CAD build for the part. Positions are in the model's coordinates, mm. A direction names the side the tool comes from. Give positions to 0.01 mm unless a question says otherwise; leave off trailing zeros. Write each loop counter-clockwise with the first axis right and the second up, starting at its lowest first coordinate (ties: lowest second). Pieces come first, ordered by that corner, then holes. Notation, with made-up numbers: (6.5, -32) - (10.5, -32) arc R13 cw to (10.5, -16) - close; hole circle Ø4 at (72.25, 53.25). An arc over 180 degrees is marked (long way). Put each result on its own line as item: value. Start each with the question number.
1. Cut at A-A on y = 28.5. List the corners of the cut face in (x, z), and give its area (3 significant figures).
2. Cut at C-C on x = -20. List the corners of the cut face in (y, z).
3. Cut at B-B on x = 28. List the corners of the cut face in (y, z).
4. Tool access for faces 5 (the flat face through (-2.5, 0, 9)), 6 (the cylindrical face through (-19.78, 36.93, 4.4)), 7 (the flat face through (-20, 0, 2.5)): list every direction of +Z, -Z, +X, -X, +Y, -Y with a clear straight run to the whole face (end or side of a thin tool).
5. Drop flat-ended pins along their axis: pin 1 (11.5 mm diameter, centred on x = -22.5, y = 2, fed in from +Z); pin 2 (6.5 mm diameter, centred on x = -20, y = 0, fed in from +Z); pin 3 (3.5 mm diameter, centred on y = 2.5, z = 10.5, fed in from -X). Give the stop position or say it passes through.
6. Mould opens along Z. For faces 1 (the cylindrical face through (-36.93, 0.5, 0.6)), 2 (the flat face through (-27, 0, 5)), 3 (the flat face through (19, -1, 8.5)), 4 (the flat face through (0, -1, 7)) say: +Z half, -Z half, draft (parallel to the pull), parting line (faces both ways), or undercut.
7. Wall check: line 1 (Z direction, x = 30.5, y = -4); line 2 (Z direction, x = -14, y = 4); line 3 (Z direction, x = -17.5, y = 1). Give the ranges that are in metal, low to high.
8. Cut at D-D on y = 0. List the corners of the cut face in (x, z).
from build123d import *

# Parameters (mm, degrees)
F0_W     = 75
F0_H     = 75
F1_DEPTH = 5
F2_W     = 40
F2_H     = 75
F3_DEPTH = 8.5
F4_W     = 75
F4_H     = 3.5
F5_DEPTH = 37.5
F6_R     = 5.25
F7_DEPTH = 2.5
F8_R     = 2


with BuildPart() as f1:
    # F0 (on Top) → F1 (new body)
    with BuildSketch(Plane.XY):
        Rectangle(F0_W, F0_H)
    extrude(amount=F1_DEPTH)

    # F2 (on face) → F3 (join)
    with BuildSketch(Plane.XY.offset(5)):
        with Locations((17.5, 0)):
            Rectangle(F2_W, F2_H)
    extrude(amount=F3_DEPTH)

    # F4 (on face) → F5 (cut, through all)
    with BuildSketch(Plane.YZ.offset(37.5)):
        with Locations((0, 6.75)):
            Rectangle(F4_W, F4_H)
    extrude(amount=-F5_DEPTH, mode=Mode.SUBTRACT)

    # F6 (on face) → F7 (cut)
    with BuildSketch(Plane.XY.offset(5)):
        with Locations((-20, 0)):
            Circle(F6_R)
    extrude(amount=-F7_DEPTH, mode=Mode.SUBTRACT)

    # F8
    f8_edges = [f1.edges().sort_by_distance(p)[0] for p in [
        (17.5, 37.5, 13.5),
        (-2.5, 0, 13.5),
        (17.5, -37.5, 13.5),
        (37.5, 0, 13.5),
        (-2.5, 37.5, 9.25),
        (-2.5, -37.5, 9.25),
        (-2.5, 0, 5),
        (-37.5, 37.5, 2.5),
        (-37.5, -37.5, 2.5),
        (-37.5, 0, 0),
        (-37.5, 0, 5),
        (0, -37.5, 0),
        (37.5, 0, 0),
        (0, 37.5, 0),
        (37.5, -37.5, 11),
        (37.5, -37.5, 2.5),
        (37.5, 37.5, 11),
        (37.5, 37.5, 2.5),
        (-20, -37.5, 5),
        (-20, 37.5, 5),
    ]]
    fillet(f8_edges, radius=F8_R)


solid = f1.part
Report:
1. outline: (-37.5, 2) arc R2 ccw to (-35.5, 0) - (35.5, 0) arc R2 ccw to (37.5, 2) - (37.5, 5) - (0, 5) - (0, 8.5) - (37.5, 8.5) - (37.5, 11.5) arc R2 ccw to (35.5, 13.5) - (-0.5, 13.5) arc R2 ccw to (-2.5, 11.5) - (-2.5, 7) arc R2 cw to (-4.5, 5) - (-35.5, 5) arc R2 ccw to (-37.5, 3) - close
1. area: 580 mm²
2. outline: (-37.5, 2) arc R2 ccw to (-35.5, 0) - (35.5, 0) arc R2 ccw to (37.5, 2) - (37.5, 3) arc R2 ccw to (35.5, 5) - (5.25, 5) - (5.25, 2.5) - (-5.25, 2.5) - (-5.25, 5) - (-35.5, 5) arc R2 ccw to (-37.5, 3) - close
3. outline: (-37.5, 2) arc R2 ccw to (-35.5, 0) - (35.5, 0) arc R2 ccw to (37.5, 2) - (37.5, 5) - (-37.5, 5) - close; (-37.5, 8.5) - (37.5, 8.5) - (37.5, 11.5) arc R2 ccw to (35.5, 13.5) - (-35.5, 13.5) arc R2 ccw to (-37.5, 11.5) - close
4. face 5: +Z, -X, +Y, -Y
4. face 6: +Z, -X, +Y
4. face 7: +Z
5. pin 1: stops at z = 5
5. pin 2: stops at z = 2.5
5. pin 3: stops at x = -2.5
6. face 1: -Z half
6. face 2: +Z half
6. face 3: undercut
6. face 4: undercut
7. line 1: z = 0 to 5, 8.5 to 13.5
7. line 2: z = 0 to 5
7. line 3: z = 0 to 2.5
8. outline: (-37.5, 2) arc R2 ccw to (-35.5, 0) - (35.5, 0) arc R2 ccw to (37.5, 2) - (37.5, 5) - (0, 5) - (0, 8.5) - (37.5, 8.5) - (37.5, 11.5) arc R2 ccw to (35.5, 13.5) - (-0.5, 13.5) arc R2 ccw to (-2.5, 11.5) - (-2.5, 7) arc R2 cw to (-4.5, 5) - (-14.75, 5) - (-14.75, 2.5) - (-25.25, 2.5) - (-25.25, 5) - (-35.5, 5) arc R2 ccw to (-37.5, 3) - close
